Geometry: final body of the model. Coordinates: model frame, mm. A direction names the side the tool comes from. Give positions to 0.01 mm unless a question says otherwise; leave off trailing zeros. Order: outer loops, then holes, each group sorted by start corner. A loop starts at its lowest first (then second) coordinate and runs counter-clockwise, first axis right, second up. Notation, with made-up numbers: (11, 13.25) -> (24, 13.25) arc R27 cw to (24, 51.25) -> close; hole circle Ø11 at (51, 6.5). An arc over 180 degrees is marked (long way). Answer in a Markdown table with one row per item. Add a question column.
Q1. Set-up query: faces 4 (the face through (28, 20, 52)), 5 (the face through (20, 40, 18)), 6 (the face through (68, 55, 48)), 7 (the face through (14, 4, 48)), 8 (the face through (68, 27, 32)). Return all of +Z, -Z, +X, -X, +Y, -Y with unobstructed straight access to the full face (end or side cutting, diameter ignored); none if empty.
Q2. Cut plane B-B on y = 10. Return the cut outline in (x, z).
Q3. Pull-direction query (Z, two-part tool) for faces 1 (the face through (32, 0, 18)), 2 (the face through (14, 8, 56)), 3 (the face through (61, 67, 64)); classes: +Z half, -Z half, draft (parallel to the pull), parting line (faces both ways), or undercut.
Q4. Cut plane A-A on z = 36.5. Return the cut outline in (x, y), and give its area (3 significant figures).
Q5. Cut plane D-D on x = 40. Return the cut outline in (y, z).
Q6. Cut plane C-C on z = 51. Return the cut outline in (x, y).
Q7. Line query: line 1 along Y through (x, z) = (9, 15); line 2 along X through (y, z) = (20, 35.5); line 3 along Y through (x, z) = (55, 50.5). Output: solid intervals per line, ascending. Write a range as from..to.
Q8. Contact query for flat-ended pins moving along their axis: P1, Ø16, axis at x = 67.5, y = 24.5, coming from the +Z side; P2, Ø3, axis at y = 44.5, z = 11.5, coming from the -X side; P3, Ø14.5, axis at x = 21, z = 32, coming from the +Y side. Output: stop coordinate, or through.
Solid Edge part; units mm, degrees
sketch "Sketch1" plane through (0, 0, 0) normal (1, 0, 0) x (0, 1, 0)
  line L0 (8, 64) -> (0, 64)
  line L1 (0, 64) -> (0, 72)
  line L2 (0, 72) -> (28, 72)
  line L3 (40, 48) -> (28, 72)
  line L4 (40, 0) -> (40, 48)
  line L5 (0, 0) -> (40, 0)
  line L6 (0, 0) -> (0, 48)
  line L7 (0, 48) -> (8, 48)
  line L8 (8, 48) -> (8, 64)
extrude "Protrusion1" add sketch "Sketch1" along normal blind 28
sketch "Sketch2" plane through (14, 0, 24) normal (0, -1, 0) x (1, 0, 0)
  line L0 (14, -24) -> (14, 8)
  line L1 (14, -24) -> (38, -24)
  line L2 (38, 8) -> (38, -24)
  arc A0 (38, 8) -> (14, 8) centre (26, 8) cw
extrude "ExtrudedProtrusion_3" add sketch "Sketch2" against normal blind 40
sketch "Sketch3" plane through (14, 0, 24) normal (0, -1, 0) x (1, 0, 0)
  line L0 (38, 8) -> (70, 8)
  arc A0 (38, -24) -> (70, 8) centre (38, 8) ccw
  line L1 (38, 8) -> (38, -24)
extrude "ExtrudedProtrusion_4" add sketch "Sketch3" against normal blind 80
sketch "Sketch4" plane through (42, 55, 24) normal (0, -1, 0) x (1, 0, 0)
  line L0 (27, 40) -> (10, 40)
  line L1 (10, 8) -> (10, 40)
  line L2 (10, 8) -> (42, 8)
  line L3 (42, 8) -> (42, 25)
  arc A0 (27, 40) -> (42, 25) centre (27, 25) cw
extrude "ExtrudedProtrusion_5" add sketch "Sketch4" against normal blind 25
Completed:
| question | item | result |
|---|---|---|
| 1 | face 4 | +Z, +X, +Y, -Y |
| 1 | face 5 | +Z, -Z, -X, +Y |
| 1 | face 6 | +Z, +X, -X, -Y |
| 1 | face 7 | +X, -X, -Y |
| 1 | face 8 | +Z, +X, -Y |
| 2 | outline | (0, 0) -> (52, 0) arc R32 ccw to (84, 32) -> (52, 32) arc R12 cw to (28, 32) -> (28, 72) -> (0, 72) -> close |
| 3 | face 1 | draft |
| 3 | face 2 | undercut |
| 3 | face 3 | +Z half |
| 4 | outline | (0, 0) -> (28, 0) -> (28, 40) -> (0, 40) -> close; (52, 55) -> (84, 55) -> (84, 80) -> (52, 80) -> close |
| 4 | area | 1,920 mm² |
| 5 | outline | (0, 0) -> (40, 0) -> (40, 20) -> (0, 20) -> close |
| 6 | outline | (0, 8) -> (28, 8) -> (28, 38.5) -> (0, 38.5) -> close; (52, 55) -> (83.87, 55) -> (83.87, 80) -> (52, 80) -> close |
| 7 | line 1 | y = 0..40 |
| 7 | line 2 | x = 0..28 |
| 7 | line 3 | y = 55..80 |
| 8 | P1 | stops at z = 32 |
| 8 | P2 | stops at x = 52 |
| 8 | P3 | stops at y = 40 |
